```python
from build123d import *

# Parameters (mm, degrees)
SKETCH1_R           = 2.7
BOSS_EXTRUDE1_DEPTH = 2
BOSS_EXTRUDE2_START = -2
BOSS_EXTRUDE2_DEPTH = 2
FILLET1_R           = 3
SKETCH2_R           = 4.375
SKETCH2_R_2         = 1.6
CUT_EXTRUDE1_DEPTH  = 84.55470457
FILLET2_R           = 10


with BuildPart() as part:
    # Sketch1 → Boss-Extrude1 (new body)
    # profile 1 of 9: a face of its own
    with BuildSketch(Plane(origin=(0, 0, 0), x_dir=(1, 0, 0), z_dir=(0, 1, 0))):
        with BuildLine():
            Line((-34.5, 20), (-34.5, -10))
            ThreePointArc((-34.5, -10), (-27.5, -17), (-20.5, -10))
            Line((-20.5, -10), (-20.5, 20))
            ThreePointArc((-20.5, 20), (-27.5, 27), (-34.5, 20))
        make_face()
        with Locations(Location((-27.5, 20, 0), (0, 0, 270))):
            Circle(SKETCH1_R, mode=Mode.SUBTRACT)
        with Locations(Location((-27.5, -10, 0), (0, 0, 270))):
            Circle(SKETCH1_R, mode=Mode.SUBTRACT)
    # profile 2 of 9: a face of its own
    with BuildSketch(Plane(origin=(0, 0, 0), x_dir=(1, 0, 0), z_dir=(0, 1, 0))):
        with BuildLine():
            ThreePointArc((-22.601020514, 25), (-21.046595612, 22.711747002), (-20.5, 20))
            Line((-20.5, 20), (-20.5, -10))
            ThreePointArc((-20.5, -10), (-27.5, -17), (-34.5, -10))
            Line((-34.5, -10), (-34.5, -50.306560208))
            ThreePointArc((-34.5, -50.306560208), (0, -61), (34.5, -50.306560208))
            Line((34.5, -50.306560208), (34.5, -10))
            ThreePointArc((34.5, -10), (27.5, -17), (20.5, -10))
            Line((20.5, -10), (20.5, 20))
            ThreePointArc((20.5, 20), (21.046595612, 22.711747002), (22.601020514, 25))
            Line((22.601020514, 25), (6.601020514, 25))
            ThreePointArc((6.601020514, 25), (0, 18.398979486), (-6.601020514, 25))
            Line((-6.601020514, 25), (-22.601020514, 25))
        make_face()
    # profile 3 of 9: a face of its own
    with BuildSketch(Plane(origin=(0, 0, 0), x_dir=(1, 0, 0), z_dir=(0, 1, 0))):
        with BuildLine():
            ThreePointArc((34.5, -10), (27.5, -17), (20.5, -10))
            Line((20.5, -10), (20.5, 20))
            ThreePointArc((20.5, 20), (27.5, 27), (34.5, 20))
            Line((34.5, 20), (34.5, -10))
        make_face()
        with Locations(Location((27.5, -10, 0), (0, 0, 270))):
            Circle(SKETCH1_R, mode=Mode.SUBTRACT)
        with Locations(Location((27.5, 20, 0), (0, 0, 270))):
            Circle(SKETCH1_R, mode=Mode.SUBTRACT)
    # profile 4 of 9: a face of its own
    with BuildSketch(Plane(origin=(0, 0, 0), x_dir=(1, 0, 0), z_dir=(0, 1, 0))):
        with BuildLine():
            ThreePointArc((-6.290744935, 27), (-6.522990426, 26.011962318), (-6.601020514, 25))
            ThreePointArc((-6.601020514, 25), (0, 18.398979486), (6.601020514, 25))
            ThreePointArc((6.601020514, 25), (6.522990426, 26.011962318), (6.290744935, 27))
            Line((6.290744935, 27), (-6.290744935, 27))
        make_face()
    # profile 5 of 9: a face of its own
    with BuildSketch(Plane(origin=(0, 0, 0), x_dir=(1, 0, 0), z_dir=(0, 1, 0))):
        with BuildLine():
            ThreePointArc((6.290744935, 27), (0, 31.601020514), (-6.290744935, 27))
            Line((-6.290744935, 27), (6.290744935, 27))
        make_face()
    # profile 6 of 9: a face of its own
    with BuildSketch(Plane(origin=(0, 0, 0), x_dir=(1, 0, 0), z_dir=(0, 1, 0))):
        with BuildLine():
            ThreePointArc((-6.290744935, 27), (-6.522990426, 26.011962318), (-6.601020514, 25))
            ThreePointArc((-6.601020514, 25), (0, 18.398979486), (6.601020514, 25))
            ThreePointArc((6.601020514, 25), (6.522990426, 26.011962318), (6.290744935, 27))
            Line((6.290744935, 27), (-6.290744935, 27))
        make_face()
    # profile 7 of 9: a face of its own
    with BuildSketch(Plane(origin=(0, 0, 0), x_dir=(1, 0, 0), z_dir=(0, 1, 0))):
        with BuildLine():
            ThreePointArc((6.290744935, 27), (0, 31.601020514), (-6.290744935, 27))
            Line((-6.290744935, 27), (6.290744935, 27))
        make_face()
    # profile 8 of 9: a face of its own
    with BuildSketch(Plane(origin=(0, 0, 0), x_dir=(1, 0, 0), z_dir=(0, 1, 0))):
        with BuildLine():
            ThreePointArc((-27.5, 27), (-24.854248689, 26.480740698), (-22.601020514, 25))
            Line((-22.601020514, 25), (-22.601020514, 27))
            Line((-22.601020514, 27), (-27.5, 27))
        make_face()
    # profile 9 of 9: a face of its own
    with BuildSketch(Plane(origin=(0, 0, 0), x_dir=(1, 0, 0), z_dir=(0, 1, 0))):
        with BuildLine():
            Line((22.601020514, 27), (22.601020514, 25))
            ThreePointArc((22.601020514, 25), (24.854248689, 26.480740698), (27.5, 27))
            Line((27.5, 27), (22.601020514, 27))
        make_face()
    extrude(amount=BOSS_EXTRUDE1_DEPTH)

    # Sketch5 → Boss-Extrude2 (add)
    with BuildSketch(Plane(origin=(0, 2, 0), x_dir=(1, 0, 0), z_dir=(0, 1, 0)).offset(BOSS_EXTRUDE2_START)):
        with BuildLine():
            Line((-55.944371359, -24.315166322), (-40, -61))
            Line((-40, -61), (0, -61))
            ThreePointArc((0, -61), (-18.059621083, -58.265342068), (-34.5, -50.306560208))
            Line((-34.5, -50.306560208), (-34.5, -13))
            ThreePointArc((-34.5, -13), (-35.964466094, -16.535533906), (-39.5, -18))
            Line((-39.5, -18), (-58.283788484, -18))
            ThreePointArc((-58.283788484, -18), (-57.201297683, -21.189892481), (-55.944371359, -24.315166322))
        make_face()
        with BuildLine():
            ThreePointArc((34.5, -50.306560208), (18.059621083, -58.265342068), (0, -61))
            Line((0, -61), (40, -61))
            Line((40, -61), (55.944371359, -24.315166322))
            ThreePointArc((55.944371359, -24.315166322), (57.201297683, -21.189892481), (58.283788484, -18))
            Line((58.283788484, -18), (39.5, -18))
            ThreePointArc((39.5, -18), (35.964466094, -16.535533906), (34.5, -13))
            Line((34.5, -13), (34.5, -50.306560208))
        make_face()
    extrude(amount=BOSS_EXTRUDE2_DEPTH)

    # Fillet1
    fillet1_edges = [part.edges().sort_by_distance(p)[0] for p in [
        (-58.283788484, 1, 18),
        (58.283788484, 1, 18),
    ]]
    fillet(fillet1_edges, radius=FILLET1_R)

    # Sketch2 → Cut-Extrude1 (cut, through all)
    with BuildSketch(Plane(origin=(0, 2, 0), x_dir=(1, 0, 0), z_dir=(0, 1, 0))):
        with Locations(Location((0, 25, 0), (0, 0, 270))):
            Circle(SKETCH2_R)
        with Locations(Location((0, -50, 0), (0, 0, 270))):
            Circle(SKETCH2_R)
        with Locations(Location((0, 0, 0), (0, 0, 270))):
            Circle(SKETCH2_R_2)
        with Locations(Location((-41.4, -30, 0), (0, 0, 270))):
            Circle(SKETCH2_R_2)
        with Locations(Location((41.4, -30, 0), (0, 0, 90))):
            Circle(SKETCH2_R_2)
    extrude(amount=-CUT_EXTRUDE1_DEPTH, mode=Mode.SUBTRACT)

    # Fillet2
    fillet2_edges = [part.edges().sort_by_distance(p)[0] for p in [
        (-40, 1, 61),
        (40, 1, 61),
    ]]
    fillet(fillet2_edges, radius=FILLET2_R)


solid = part.part
```
Check sheet for the modelled part. Datum: model origin and axes. Units: mm. Give positions to 0.01 mm unless a question says otherwise; leave off trailing zeros. Write each loop counter-clockwise with the first axis right and the second up, starting at its lowest first coordinate (ties: lowest second). Pieces come first, ordered by that corner, then holes.
Item 1: Scan lines: L1, parallel to X at y = 1.2, z = 10; L2, parallel to Z at x = -1, y = 0.3; L3, parallel to X at y = 0.9, z = -5. Record each from-to range of solid material in increasing order.
Item 2: Cross-section at D-D (y = 0.85). Count the separate pieces of the cut face and the enclosed holes in it, and give its area (3 significant figures).
Item 3: Gauge pin test, flat ends, axial feed: pin 1 (0.6 mm diameter, centred on x = 24.5, y = 0.5, fed in from -Z); pin 2 (1 mm diameter, centred on y = 1.5, z = -10, fed in from -X); pin 3 (1 mm diameter, centred on x = 16, y = 2, fed in from -Z). Record the tip position at first contact, or that the pin passes through.
Item 4: Cross-section at B-B (z = 30). Enter the section's corners in (x, y).
Item 5: Cross-section at A-A (x = 0). Enter the section's corners in (y, z) (3 decimals), and give its area (3 significant figures).
Item 6: Cross-section at C-C (x = -41.4). Enter the section's corners in (y, z), and give its area (3 significant figures).
Item 7: Draft check along Z on faces 1 (the face through (-56.517, 1.014, 19.272)), 2 (the face through (36, 0.99, 16.57)), 3 (the face through (-24.823, 0.986, -20.351)). Enter one of: released by +Z, released by -Z, zero draft, split by the parting line, or undercut.
Report:
1. L1: x = -34.5 to -30.2, -24.8 to 24.8, 30.2 to 34.5
1. L2: z = -31.52 to -29.26, -20.74 to -1.25, 1.25 to 45.74, 54.26 to 61
1. L3: x = -34.5 to 34.5
2. separate pieces: 1
2. enclosed holes: 9
2. area: 7,060 mm2
3. pin 1: stops at z = -27
3. pin 2: stops at x = -34.5
3. pin 3: stops at z = -25
4. outline: (-53.47, 0) - (-43, 0) - (-43, 2) - (-53.47, 2) - close; (-39.8, 0) - (39.8, 0) - (39.8, 2) - (-39.8, 2) - close; (43, 0) - (53.47, 0) - (53.47, 2) - (43, 2) - close
5. outline: (0, -31.601) - (2, -31.601) - (2, -29.375) - (0, -29.375) - close; (0, -20.625) - (2, -20.625) - (2, -1.6) - (0, -1.6) - close; (0, 1.6) - (2, 1.6) - (2, 45.625) - (0, 45.625) - close; (0, 54.375) - (2, 54.375) - (2, 61) - (0, 61) - close
5. area: 144 mm2
6. outline: (0, 18) - (2, 18) - (2, 28.4) - (0, 28.4) - close; (0, 31.6) - (2, 31.6) - (2, 57.06) - (0, 57.06) - close
6. area: 71.7 mm2
7. face 1: split by the parting line
7. face 2: released by -Z
7. face 3: undercut
